Could you check a few things on this drawing? It's one solid part, dimensions in mm from its lowest x, y, z. Round coordinates to 2 decimals unless told otherwise and drop trailing zeros. Write each loop counter-clockwise with the first axis right and the second up, starting at its lowest first coordinate (ties: lowest second). Pieces come first, ordered by that corner, then holes. Notation, with made-up numbers: (-30.5, -7) -> (-11.5, -7) arc R27 ccw to (-11.5, 16) -> close; hole circle Ø7 at (51.25, 62.5). An arc over 180 degrees is marked (long way). Answer in a Markdown table with one row per item.
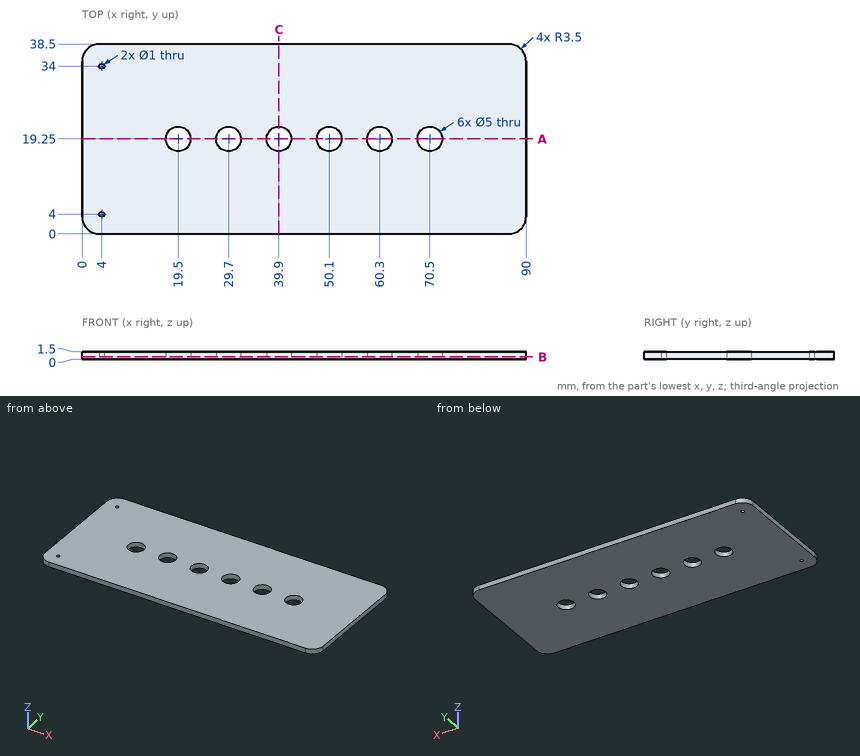
1) I want a section at C-C, the plane x = 39.9. List the corners of the cut face in (y, z) for me, and give its area (4 significant figures).
Response:
| item | result |
|---|---|
| outline | (0, 0) -> (16.75, 0) -> (16.75, 1.5) -> (0, 1.5) -> close; (21.75, 0) -> (38.5, 0) -> (38.5, 1.5) -> (21.75, 1.5) -> close |
| area | 50.25 mm^2 |
2) I need wall thicknesses on line 1 (Y direction, x = 4, z = 0.6); line 2 (X direction, y = 34, z = 0.4); line 3 (Y direction, x = 40, z = 1.4). Which ranges of each line are inside material? Lowest first, please. Write a range as [from, to].
Response:
| item | result |
|---|---|
| line 1 | y = [0, 3.5], [4.5, 33.5], [34.5, 38.5] |
| line 2 | x = [0, 3.5], [4.5, 90] |
| line 3 | y = [0, 16.75], [21.75, 38.5] |
3) For pin 1 (4.5 mm diameter, centred on x = 70.5, y = 19.25, fed in from -Z), with a flat end and sliding along its axis, tell me the tip position at first contact or that it passes through.
Response:
| item | result |
|---|---|
| pin 1 | passes through |
4) I want a section at B-B, the plane z = 0.5. Count the separate pieces of the cut face and the enclosed holes in it, and give its area (3 significant figures).
Response:
| item | result |
|---|---|
| separate pieces | 1 |
| enclosed holes | 8 |
| area | 3,340 mm^2 |
5) I want a section at A-A, the plane y = 19.25. List the corners of the cut face in (x, z) for me.
Response:
| item | result |
|---|---|
| outline | (0, 0) -> (17, 0) -> (17, 1.5) -> (0, 1.5) -> close; (22, 0) -> (27.2, 0) -> (27.2, 1.5) -> (22, 1.5) -> close; (32.2, 0) -> (37.4, 0) -> (37.4, 1.5) -> (32.2, 1.5) -> close; (42.4, 0) -> (47.6, 0) -> (47.6, 1.5) -> (42.4, 1.5) -> close; (52.6, 0) -> (57.8, 0) -> (57.8, 1.5) -> (52.6, 1.5) -> close; (62.8, 0) -> (68, 0) -> (68, 1.5) -> (62.8, 1.5) -> close; (73, 0) -> (90, 0) -> (90, 1.5) -> (73, 1.5) -> close |
